from build123d import *

# Parameters (mm, degrees)
CROQUIS1_R              = 2
SALIENTE_EXTRUIR1_DEPTH = 3


with BuildPart() as part:
    # Croquis1 → Saliente-Extruir1 (new body)
    with BuildSketch(Plane.XY):
        with BuildLine():
            Line((40, 0), (40, -47))
            Line((40, -47), (20.175, -47))
            Line((20.175, -47), (20.175, -50.2))
            Line((20.175, -50.2), (-20.175, -50.2))
            Line((-20.175, -50.2), (-20.175, -47))
            Line((-20.175, -47), (-40, -47))
            Line((-40, -47), (-40, 0))
            ThreePointArc((-40, 0), (-28.284271247, 28.284271247), (0, 40))
            ThreePointArc((0, 40), (28.284271247, 28.284271247), (40, 0))
        make_face()
        with Locations((-30, -11.85)):
            Circle(CROQUIS1_R, mode=Mode.SUBTRACT)
        with Locations(Location((30, -11.85, 0), (0, 0, 180))):
            Circle(CROQUIS1_R, mode=Mode.SUBTRACT)
        Circle(CROQUIS1_R, mode=Mode.SUBTRACT)
    extrude(amount=SALIENTE_EXTRUIR1_DEPTH)


solid = part.part
The listing builds one solid part. Answer for the finished solid, in the listing's coordinates (mm). A direction names the side the tool comes from. Coordinates: 2 decimals unless noted, no trailing zeros. Write each loop counter-clockwise with the first axis right and the second up, starting at its lowest first coordinate (ties: lowest second). Pieces come first, ordered by that corner, then holes. Notation, with made-up numbers: (69, -16.75) - (81, -16.75) arc R37 cw to (81, 20.25) - close; hole circle Ø4 at (9.25, -29.75). An arc over 180 degrees is marked (long way). Answer as CSV lines item,"result".
1. Straight lines are drawn through the part: line 1 (X direction, y = -1, z = 1.85); line 2 (Y direction, x = -0.5, z = 0.95); line 3 (Y direction, x = 30, z = 1.45). For each, find the intervals that lie inside material, in ascending order. Write a range as [from, to].
Computed values:
line 1,"x = [-40, -1.73], [1.73, 40]"
line 2,"y = [-50.2, -1.94], [1.94, 40]"
line 3,"y = [-47, -13.85], [-9.85, 26.46]"
2. A tool of negligible diameter and unlimited length cuts with its end or side. For faces 1 (the flat face through (1, -4, 3)), 2 (the flat face through (-30, -47, 1)), 3 (the flat face through (30, -47, 1)), from which of +Z, -Z, +X, -X, +Y, -Y can it reach the whole face along a straight path? Write none if from no direction.
Computed values:
face 1,"+Z, +X, -X, +Y, -Y"
face 2,"+Z, -Z, -X, -Y"
face 3,"+Z, -Z, +X, -Y"
3. Find section B-B (z = 2.45). Give the vertices of the cut face in (x, y) (3 decimals).
Computed values:
outline,"(-40, -47) - (-20.175, -47) - (-20.175, -50.2) - (20.175, -50.2) - (20.175, -47) - (40, -47) - (40, 0) arc R40 ccw to (-40, 0) - close; hole circle Ø4 at (-30, -11.85); hole circle Ø4 at (0, 0); hole circle Ø4 at (30, -11.85)"
4. Find section C-C (y = 1). Give the vertices of the cut face in (x, z), plus the area to 3 significant figures.
Computed values:
outline,"(-39.99, 0) - (-1.73, 0) - (-1.73, 3) - (-39.99, 3) - close; (1.73, 0) - (39.99, 0) - (39.99, 3) - (1.73, 3) - close"
area,"230 mm²"
5. Given P1, Ø1.5, axis at x = -18, z = 1, coming from the +Y side; P2, Ø1.5, axis at y = -49, z = 1.5, coming from the -X side (3 decimals); P3, Ø1.5, axis at y = 14.5, z = 1, coming from the +X side, each flat-ended and moving along its own axis, determine where each tip first touches the part or whether it passes through.
Computed values:
P1,"stops at y = 36.09"
P2,"stops at x = -20.175"
P3,"stops at x = 37.56"
6. Find section A-A (y = -11.85). Give the vertices of the cut face in (x, z).
Computed values:
outline,"(-40, 0) - (-32, 0) - (-32, 3) - (-40, 3) - close; (-28, 0) - (28, 0) - (28, 3) - (-28, 3) - close; (32, 0) - (40, 0) - (40, 3) - (32, 3) - close"
7. Find section D-D (x = -30). Give the vertices of the cut face in (y, z).
Computed values:
outline,"(-47, 0) - (-13.85, 0) - (-13.85, 3) - (-47, 3) - close; (-9.85, 0) - (26.46, 0) - (26.46, 3) - (-9.85, 3) - close"
8. Determine the mould class of faces 4 (the flat face through (40, -23, 1)), 5 (the cylindrical face through (0, -2, 1)), 6 (the flat face through (0, -50.2, 1)), 7 (the flat face through (-20.175, -49, 1)) for opening direction X: +X half, -X half, draft (parallel to the pull), parting line (faces both ways), or undercut.
Computed values:
face 4,"+X half"
face 5,"undercut"
face 6,"draft"
face 7,"-X half"
